from build123d import *

# Parameters (mm, degrees)
SKETCH1_R               = 5.05
SKETCH1_R_2             = 3.05
BOSS_EXTRUDE1_DEPTH     = 11
BOSS_EXTRUDE2_START     = 11
SKETCH1_3_R             = 5.05
SKETCH1_3_R_2           = 3.05
SKETCH1_3_R_3           = 2
BOSS_EXTRUDE2_DEPTH     = 2
CUT_EXTRUDE1_REACH      = 16.833
CUT_EXTRUDE1_END_RADIUS = 5.05
SKETCH2_R               = 1.6
CHAMFER1_SIZE           = 1.2


with BuildPart() as part:
    # Sketch1 → Boss-Extrude1 (new body)
    with BuildSketch(Plane(origin=(0, 0, 0), x_dir=(0, 1, 0), z_dir=(0, 0, 1))):
        with Locations(Location((0, 0, 0), (0, 0, 270))):
            Circle(SKETCH1_R)
        with Locations(Location((0, 0, 0), (0, 0, 270))):
            Circle(SKETCH1_R_2, mode=Mode.SUBTRACT)
    extrude(amount=BOSS_EXTRUDE1_DEPTH)

    # Sketch1<3> → Boss-Extrude2 (add)
    # profile 1 of 2: a face of its own
    with BuildSketch(Plane(origin=(0, 0, 0), x_dir=(0, 1, 0), z_dir=(0, 0, 1)).offset(BOSS_EXTRUDE2_START)):
        with Locations(Location((0, 0, 0), (0, 0, 270))):
            Circle(SKETCH1_3_R)
        with Locations(Location((0, 0, 0), (0, 0, 270))):
            Circle(SKETCH1_3_R_2, mode=Mode.SUBTRACT)
    # profile 2 of 2: a face of its own
    with BuildSketch(Plane(origin=(0, 0, 0), x_dir=(0, 1, 0), z_dir=(0, 0, 1)).offset(BOSS_EXTRUDE2_START)):
        with Locations(Location((0, 0, 0), (0, 0, 270))):
            Circle(SKETCH1_3_R_2)
        with Locations(Location((0, 0, 0), (0, 0, 270))):
            Circle(SKETCH1_3_R_3, mode=Mode.SUBTRACT)
    extrude(amount=BOSS_EXTRUDE2_DEPTH)

    # Cut-Extrude1: up to this cylinder (the profile starts inside it)
    cut_extrude1_end = Plane(origin=(0, 0, 3), z_dir=(0, 0, -1)) * Cylinder(CUT_EXTRUDE1_END_RADIUS, 44.766, mode=Mode.PRIVATE)
    # Sketch2 → Cut-Extrude1 (cut, up to the surface)
    with BuildSketch(Plane(origin=(0, 0, 0), x_dir=(-1, 0, 0), z_dir=(0, 1, 0)), mode=Mode.PRIVATE) as cut_extrude1_sk1:
        with Locations(Location((0, 3, 0), (0, 0, 90))):
            Circle(SKETCH2_R)
    cut_extrude1_tool1 = extrude(cut_extrude1_sk1.sketch, amount=-CUT_EXTRUDE1_REACH, mode=Mode.PRIVATE) & cut_extrude1_end
    add(cut_extrude1_tool1.solids().sort_by_distance((0, 0, 3))[0], mode=Mode.SUBTRACT)

    # Chamfer1
    # the kernel refuses this chamfer: 1.2 mm, written as the material it adds along each edge
    with BuildSketch(Plane(origin=(0, 0, 11), x_dir=(1, 0, 0), z_dir=(0, -1, 0))) as chamfer1_piece_1_section:
        Polygon((3.05, -CHAMFER1_SIZE), (3.05 - CHAMFER1_SIZE, 0), (3.05, 0), align=None)
    chamfer1_piece_1 = revolve(axis=Axis((0, 0, 11), (0, 0, 1)), mode=Mode.PRIVATE)
    chamfer1_piece_1 = chamfer1_piece_1 - Plane(origin=(0, 0, 10.324643315), x_dir=(1, 0, 0), z_dir=(0, 0, -1)) * Cylinder(2, 13, mode=Mode.PRIVATE)
    add(chamfer1_piece_1)


solid = part.part
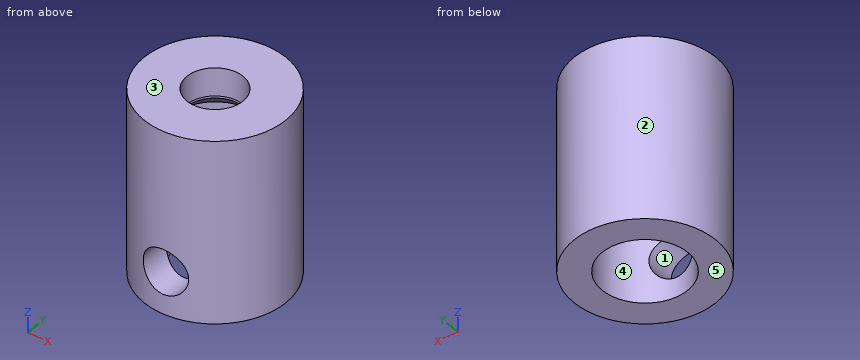
Design review of the part built by this model. Coordinates are the model's own, in mm. Face numbers are marked on the shaded views. A direction names the side the tool comes from. Give positions to 0.01 mm unless a question says otherwise; leave off trailing zeros. Order: outer loops, then holes, each group sorted by start corner. A loop starts at its lowest first (then second) coordinate and runs counter-clockwise, first axis right, second up.
1. Add section A-A, the plane y = 0. State the section outline as (x, z) points, then the cut area to 3 significant figures.
Solution:
outline: (-5.05, 0) - (-3.05, 0) - (-3.05, 9.8) - (-2, 10.85) - (-2, 13) - (-5.05, 13) - close; (2, 10.85) - (3.05, 9.8) - (3.05, 0) - (5.05, 0) - (5.05, 13) - (2, 13) - close
area: 57.6 mm2
2. To check wall thickness, follow L1, parallel to Y at x = 0, z = 11; L2, parallel to Z at x = 0, y = -4.25; L3, parallel to Y at x = 0, z = 4. State the ranges of each line that lie inside material, in increasing order.
Solution:
L1: y = -5.05 to -2, 2 to 5.05
L2: z = 0 to 1.4, 4.6 to 13
L3: y = 3.05 to 5.05
3. Add section B-B, the plane x = 0. State the section outline as (y, z) points, then the cut area to 3 significant figures.
Solution:
outline: (-5.05, 0) - (-3.05, 0) - (-3.05, 1.4) - (-5.05, 1.4) - close; (-5.05, 4.6) - (-3.05, 4.6) - (-3.05, 9.8) - (-2, 10.85) - (-2, 13) - (-5.05, 13) - close; (2, 10.85) - (3.05, 9.8) - (3.05, 0) - (5.05, 0) - (5.05, 13) - (2, 13) - close
area: 51.2 mm2
4. Add section C-C, the plane z = 5.5. State the section outline as (x, y) points, then the cut area to 3 significant figures.
Solution:
outline: circle Ø10.1 at (0, 0); hole circle Ø6.1 at (0, 0)
area: 50.9 mm2
5. For pin 1 Ø5 at (x, y) = (0, 0) entering from -Z; pin 2 Ø2 at (y, z) = (-4, 6.5) entering from -X; pin 3 Ø5 at (x, z) = (-3.5, 2.5) entering from -Y, all flat-tipped, find the tip position at first contact; note any pin that passes through.
Solution:
pin 1: stops at z = 10.35
pin 2: stops at x = -4.06
pin 3: stops at y = -4.93
6. Tool access review of the marked faces 4 and 5: name each direction out of +Z, -Z, +X, -X, +Y, -Y from which nothing blocks a thin tool from reaching the whole face with its end or side.
Solution:
face 4: -Z
face 5: -Z, +X, -X, +Y, -Y
7. Add section D-D, the plane y = -4.5. State the section outline as (x, z) points, then the cut area to 3 significant figures.
Solution:
outline: (-2.29, 0) - (2.29, 0) - (2.29, 13) - (-2.29, 13) - close; hole circle Ø3.2 at (0, 3)
area: 51.5 mm2
8. Mouldability with a two-part tool opening along X and no side actions: class the marked faces 1, 2 and 3 as +X half, -X half, draft (parallel to the pull), parting line (faces both ways), or undercut.
Solution:
face 1: undercut
face 2: parting line
face 3: draft
